For this review, take the finished solid that the model builds, in its own axes (mm). A direction names the side the tool comes from. Round coordinates to 2 decimals unless told otherwise and drop trailing zeros. Write each loop counter-clockwise with the first axis right and the second up, starting at its lowest first coordinate (ties: lowest second). Pieces come first, ordered by that corner, then holes. Notation, with made-up numbers: (15.25, -39.75) - (33.25, -39.75) arc R20 cw to (33.25, -15.75) - close; hole circle Ø5 at (61, -19). An arc over 180 degrees is marked (long way). One line per item, written item: value. Start each with the question number.
Q1. Clearance check with flat-ended pins moving along their axes: pin 1 Ø1 at (x, z) = (1, 21.5) entering from -Y; pin 2 Ø3 at (x, y) = (-24, -0.85) entering from -Z; pin 3 Ø6 at (y, z) = (-9.5, 11) entering from -X; pin 4 Ø2.5 at (x, z) = (-24.5, 9.5) entering from -Y. State where each tip first meets the part, or that it passes through.
Q2. Add section C-C on y = 8.75. Write out the cut boundary in (x, z), and give its area (3 significant figures).
Q3. Mouldability with a two-part tool opening along X and no side actions: class faces 1 (the face through (11, 4, 5)), 2 (the face through (23.986, 11.056, 19.297)), 3 (the face through (-0.1, 1.3, 14)) as +X half, -X half, draft (parallel to the pull), parting line (faces both ways), or undercut.
Q4. Tool access review of faces 4 (the face through (23.5, 1.3, 14)), 5 (the face through (-30, 0, 6)), 6 (the face through (-24.297, 11.056, 18.986)), 7 (the face through (11, -6, 5)), 8 (the face through (29, 7, 12)): name each direction out of +Z, -Z, +X, -X, +Y, -Y from which nothing blocks a thin tool from reaching the whole face with its end or side.
Q5. Add section D-D on z = 10.25. Give the number of separate pieces and of enclosed holes in the cut face, and give its area (3 significant figures).
Q6. Add section A-A on y = -0.85. Write out the cut boundary in (x, z).
Q7. Add section B-B on x = 25. Write out the cut boundary in (y, z), and give its area (3 significant figures).
Q8. For probe 1 along X at (y, z) = (-4.65, 13); probe 2 along Y at (x, z) = (0, 9.5); probe 3 along X at (y, z) = (6, 5.75), list the stretches that pass through material, from the lowest coordinate up.
```python
from build123d import *

# Parameters (mm, degrees)
SCHIZZO1_W                   = 60
SCHIZZO1_H                   = 30
ESTRUSIONE_ESTRUSIONE1_DEPTH = 5
SCHIZZO2_W                   = 60
SCHIZZO2_H                   = 8
ESTRUSIONE_ESTRUSIONE2_DEPTH = 20
SCHIZZO3_R                   = 5
TAGLIO_ESTRUSIONE1_DEPTH     = 8
RACCORDO1_R                  = 20
SCHIZZO4_W                   = 60
SCHIZZO4_H                   = 15
ESTRUSIONE_ESTRUSIONE3_DEPTH = 10
SCHIZZO6_R                   = 8
TAGLIO_ESTRUSIONE2_DEPTH     = 15
SCHIZZO8_W                   = 60
SCHIZZO8_H                   = 4.7
ESTRUSIONE_ESTRUSIONE4_DEPTH = 10
SCHIZZO9_R                   = 6.3
TAGLIO_ESTRUSIONE3_DEPTH     = 5
SCHIZZO10_R                  = 2
TAGLIO_ESTRUSIONE4_DEPTH     = 16
SCHIZZO11_W                  = 60
SCHIZZO11_H                  = 15
TAGLIO_ESTRUSIONE5_DEPTH     = 1


with BuildPart() as part:
    # Schizzo1 → Estrusione-Estrusione1 (new body)
    with BuildSketch(Plane.XY):
        Rectangle(SCHIZZO1_W, SCHIZZO1_H)
    extrude(amount=ESTRUSIONE_ESTRUSIONE1_DEPTH)

    # Schizzo2 → Estrusione-Estrusione2 (add)
    with BuildSketch(Plane.XY.offset(5)):
        with Locations((0, 11)):
            Rectangle(SCHIZZO2_W, SCHIZZO2_H)
    extrude(amount=ESTRUSIONE_ESTRUSIONE2_DEPTH)

    # Schizzo3 → Taglio-Estrusione1 (cut)
    with BuildSketch(Plane(origin=(0, 15, 0), x_dir=(1, 0, 0), z_dir=(0, 1, 0))):
        with Locations((11, -13)):
            Circle(SCHIZZO3_R)
        with Locations((-11, -13)):
            Circle(SCHIZZO3_R)
    extrude(amount=-TAGLIO_ESTRUSIONE1_DEPTH, mode=Mode.SUBTRACT)

    # Raccordo1
    raccordo1_edges = [part.edges().sort_by_distance(p)[0] for p in [
        (30, 11, 25),
        (-30, 11, 25),
    ]]
    fillet(raccordo1_edges, radius=RACCORDO1_R)

    # Schizzo4 → Estrusione-Estrusione3 (add)
    with BuildSketch(Plane.XY.offset(5)):
        with Locations((0, -0.5)):
            Rectangle(SCHIZZO4_W, SCHIZZO4_H)
    extrude(amount=ESTRUSIONE_ESTRUSIONE3_DEPTH)

    # Schizzo6 → Taglio-Estrusione2 (cut)
    with BuildSketch(Plane.XZ.offset(8)):
        with Locations((-11, 13)):
            Circle(SCHIZZO6_R)
        with Locations((11, 13)):
            Circle(SCHIZZO6_R)
    extrude(amount=-TAGLIO_ESTRUSIONE2_DEPTH, mode=Mode.SUBTRACT)

    # Schizzo8 → Estrusione-Estrusione4 (add)
    with BuildSketch(Plane.XY.offset(15)):
        with Locations((0, -0.85)):
            Rectangle(SCHIZZO8_W, SCHIZZO8_H)
    extrude(amount=-ESTRUSIONE_ESTRUSIONE4_DEPTH)

    # Schizzo9 → Taglio-Estrusione3 (cut)
    with BuildSketch(Plane.XZ.offset(3.2)):
        with Locations((-11, 13)):
            Circle(SCHIZZO9_R)
        with Locations((11, 13)):
            Circle(SCHIZZO9_R)
    extrude(amount=-TAGLIO_ESTRUSIONE3_DEPTH, mode=Mode.SUBTRACT)

    # Schizzo10 → Taglio-Estrusione4 (cut, through all)
    with BuildSketch(Plane.XY.offset(15)):
        with Locations((0, -0.85)):
            Circle(SCHIZZO10_R)
        with Locations((24, -0.85)):
            Circle(SCHIZZO10_R)
        with Locations((-24, -0.85)):
            Circle(SCHIZZO10_R)
    extrude(amount=-TAGLIO_ESTRUSIONE4_DEPTH, mode=Mode.SUBTRACT)

    # Schizzo11 → Taglio-Estrusione5 (cut)
    with BuildSketch(Plane.XY.offset(15)):
        with Locations((0, -0.5)):
            Rectangle(SCHIZZO11_W, SCHIZZO11_H)
    extrude(amount=-TAGLIO_ESTRUSIONE5_DEPTH, mode=Mode.SUBTRACT)


solid = part.part
```
Result set:
1. pin 1: stops at y = 7
1. pin 2: passes through
1. pin 3: stops at x = -30
1. pin 4: stops at y = -8
2. outline: (-30, 0) - (30, 0) - (30, 5) arc R20 ccw to (10, 25) - (-10, 25) arc R20 ccw to (-30, 5) - close; hole circle Ø10 at (-11, 13); hole circle Ø10 at (11, 13)
2. area: 1,170 mm^2
3. face 1: undercut
3. face 2: +X half
3. face 3: draft
4. face 4: +Z, +X, -X, -Y
4. face 5: +Z, -Z, -X, +Y, -Y
4. face 6: +Z, -X, +Y
4. face 7: -Y
4. face 8: +Z, +X, +Y
5. separate pieces: 3
5. enclosed holes: 3
5. area: 781 mm^2
6. outline: (-30, 0) - (-26, 0) - (-26, 14) - (-30, 14) - close; (-22, 0) - (-2, 0) - (-2, 14) - (-4.78, 14) arc R6.3 cw (long way) to (-17.22, 14) - (-22, 14) - close; (2, 0) - (22, 0) - (22, 14) - (17.22, 14) arc R6.3 cw (long way) to (4.78, 14) - (2, 14) - close; (26, 0) - (30, 0) - (30, 14) - (26, 14) - close
7. outline: (-15, 0) - (-2.58, 0) - (-2.58, 14) - (-8, 14) - (-8, 5) - (-15, 5) - close; (0.88, 0) - (15, 0) - (15, 18.23) - (7, 18.23) - (7, 14) - (0.88, 14) - close
7. area: 342 mm^2
8. probe 1: x = -30 to -19, -3 to 3, 19 to 30
8. probe 2: y = -8 to -2.85, 1.15 to 15
8. probe 3: x = -30 to -14.38, -7.62 to 7.62, 14.38 to 30
